from build123d import *

# Parameters (mm, degrees)
F0_R      = 4.7625
F2_R      = 4.7625
F5_FACE_R = 4.7625
F4_W      = 3.175
F4_H      = 3.175
F9_W      = 3.175
F9_H      = 3.175
F8_W      = 0.79375
F8_H      = 0.79375
F11_R     = 2.6419390303
F12_DEPTH = 0.1984375


with BuildPart() as f5:
    # F0 (on Top) → F5 section 0
    with BuildSketch(Plane.XY):
        Circle(F0_R)
    # F2 (on offset) → F5 section 1
    with BuildSketch(Plane.XY.offset(1.5875)):
        Circle(F2_R)
    loft()

    # F5_face (on face) → F6 section 0
    with BuildSketch(Plane.XY.offset(1.5875)):
        Circle(F5_FACE_R)
    # F4 (on offset) → F6 section 1
    with BuildSketch(Plane.XY.offset(3.175)):
        Rectangle(F4_W, F4_H)
    loft()

    # F9 (on face) → F10 section 0
    with BuildSketch(Plane(origin=(0, 0, 0), x_dir=(1, 0, 0), z_dir=(0, 0, -1))):
        Rectangle(F9_W, F9_H)
    # F8 (on offset) → F10 section 1
    with BuildSketch(Plane.XY.offset(-31.496)):
        Rectangle(F8_W, F8_H)
    loft()

    # F11 (on offset) → F12 (cut)
    with BuildSketch(Plane.XY.offset(3.175)):
        Circle(F11_R)
    extrude(amount=-F12_DEPTH, mode=Mode.SUBTRACT)


solid = f5.part
Geometry: final body of the model. Coordinates: model frame, mm. A direction names the side the tool comes from. Coordinates: 2 decimals unless noted, no trailing zeros.
(1) Access query for faces 1 (the face through (-3.78, -2.9, 0.8)), 2 (the face through (2, 0, 0)). Directions: +Z, -Z, +X, -X, +Y, -Y. A direction counts if a zero-diameter tool reaches every point of the face in a straight line with its end or side. Return the directions, or none.
(2) First-contact query: pin 1 (5 mm diameter, centred on x = -3, z = -17.5, fed in from +Y); pin 2 (1.5 mm diameter, centred on x = 2, y = -3, fed in from +Z); pin 3 (4 mm diameter, centred on x = -1, z = -26, fed in from +Y). Flat tips, straight axial feed; report the tip coordinate or a pass-through.
(3) Material intervals for probe 1 along Z at (x, y) = (-2.5, -0.5); probe 2 along X at (y, z) = (0, -9.5); probe 3 along Z at (x, y) = (-3.75, -0.75), sorted ascending.
Solution:
1. face 1: +Z, -Z
1. face 2: -Z
2. pin 1: stops at y = 0.98
2. pin 2: stops at z = 2.68
2. pin 3: stops at y = 0.68
3. probe 1: z = 0 to 2.71
3. probe 2: x = -1.23 to 1.23
3. probe 3: z = 0 to 2.06
